Check sheet for the modelled part. Datum: model origin and axes. Units: mm. A direction names the side the tool comes from. Round coordinates to 2 decimals unless told otherwise and drop trailing zeros. Loops run counter-clockwise (first coordinate to the right, second up) from the corner with the lowest first, then second, coordinate; pieces in that order, holes last. Notation, with made-up numbers: (-8, -11) - (45, -11) arc R20 ccw to (45, -5) - close; hole circle Ø3 at (10.5, 30). An arc over 180 degrees is marked (long way). Put each result on its own line as item: value.
```python
from build123d import *

# Parameters (mm, degrees)
F0_R      = 17.4625
F0_R_2    = 4.7625
F1_DEPTH  = 4.7752
F2_R      = 7.9375
F2_R_2    = 4.7625
F3_DEPTH  = 6.35
F5_R      = 1.5875
F6_DEPTH  = 4.7762
F8_R      = 1.4224
F9_DEPTH  = 5.08
F11_R     = 1.4224
F12_DEPTH = 5.08


with BuildPart() as f1:
    # F0 (on Front) → F1 (new body)
    with BuildSketch(Plane.XZ):
        Circle(F0_R)
        Circle(F0_R_2, mode=Mode.SUBTRACT)
    extrude(amount=F1_DEPTH)

    # F2 (on face) → F3 (join)
    with BuildSketch(Plane.XZ.offset(4.7752)):
        Circle(F2_R)
        Circle(F2_R_2, mode=Mode.SUBTRACT)
    extrude(amount=F3_DEPTH)

    # F5 (on face) → F6 (cut, through all)
    with BuildSketch(Plane.XZ.offset(4.7752)):
        with Locations((0, 13.97)):
            Circle(F5_R)
    extrude(amount=-F6_DEPTH, mode=Mode.SUBTRACT)

    # F8 (on offset) → F9 (cut)
    with BuildSketch(Plane.XY.offset(7.9375)):
        with Locations((0, -7.9502)):
            Circle(F8_R)
    extrude(amount=-F9_DEPTH, mode=Mode.SUBTRACT)

    # F11 (on offset) → F12 (cut)
    with BuildSketch(Plane.YZ.offset(7.9375)):
        with Locations((-7.9502, 0)):
            Circle(F11_R)
    extrude(amount=-F12_DEPTH, mode=Mode.SUBTRACT)


solid = f1.part
```
Item 1: Section check A-A on z = 0. Enter the section's corners in (x, y).
Filled sheet:
outline: (-17.46, -4.78) - (-7.94, -4.78) - (-7.94, -11.13) - (-4.76, -11.13) - (-4.76, 0) - (-17.46, 0) - close; (4.76, -11.13) - (7.94, -11.13) - (7.94, -9.37) - (4.76, -9.37) - close; (4.76, -6.53) - (7.94, -6.53) - (7.94, -4.78) - (17.46, -4.78) - (17.46, 0) - (4.76, 0) - close
Item 2: Section check D-D on z = 13.97. Enter the section's corners in (x, y).
Filled sheet:
outline: (-10.48, -4.78) - (-1.59, -4.78) - (-1.59, 0) - (-10.48, 0) - close; (1.59, -4.78) - (10.48, -4.78) - (10.48, 0) - (1.59, 0) - close
Item 3: Release check for a two-part mould opening along X. For faces 4 (the cylindrical face through (-1.03, -5.48, -4.65)), 5 (the flat face through (0, -11.125, -5)), 6 (the cylindrical face through (-1.72, -7.91, -7.75)) record: +X half, -X half, draft (parallel to the pull), parting line (faces both ways), or undercut.
Filled sheet:
face 4: undercut
face 5: draft
face 6: parting line
Item 4: Tool access check on faces 1 (the flat face through (4, -4.775, -8)), 2 (the cylindrical face through (1.314, -8.495, 6.262)), 3 (the cylindrical face through (6.265, -6.593, 0.427)). Record the directions out of +Z, -Z, +X, -X, +Y, -Y that give a thin tool (end or side, any length) a straight path to the whole face; none if there is none.
Filled sheet:
face 1: -Y
face 2: +Z
face 3: +X
Item 5: Thickness scan on line 1 (Z direction, x = 0, y = -2.55); line 2 (Z direction, x = 0, y = -5); line 3 (Y direction, x = 0, z = 5.4). Record the ranges inside material, lowest first. Write a range as from..to.
Filled sheet:
line 1: -17.46..-4.76, 4.76..12.38, 15.56..17.46
line 2: -7.94..-4.76, 4.76..7.94
line 3: -11.13..-9.37, -6.53..0
Item 6: Go/stop test with flat-tipped pins: pin 1 (3 mm diameter, centred on x = 10.5, z = 6, fed in from -Y); pin 2 (3 mm diameter, centred on y = -4.5, z = 8, fed in from -X); pin 3 (6 mm diameter, centred on x = 13, y = -6.5, fed in from +Z); pin 4 (10.5 mm diameter, centred on x = -0.5, z = 1.5, fed in from -Y). Record where each tip stops, or that it passes through.
Filled sheet:
pin 1: y = -4.78
pin 2: x = -16.21
pin 3: z = 13.92
pin 4: y = -11.13
Item 7: Section check B-B on x = 2. Enter the section's corners in (y, z), then the cut area to 3 significant figures.
Filled sheet:
outline: (-11.13, -7.68) - (-4.78, -7.68) - (-4.78, -17.35) - (0, -17.35) - (0, -4.32) - (-11.13, -4.32) - close; (-11.13, 4.32) - (0, 4.32) - (0, 17.35) - (-4.78, 17.35) - (-4.78, 7.68) - (-11.13, 7.68) - close
area: 167 mm²
Item 8: Section check C-C on y = -8.5. Enter the section's corners in (x, z) (1 decimal).
Filled sheet:
outline: (-1.3, 4.6) - (-1.3, 7.8) arc R7.9 ccw (long way) to (7.8, -1.3) - (4.6, -1.3) arc R4.8 cw (long way) to start; (1.3, 4.6) arc R4.8 cw to (4.6, 1.3) - (7.8, 1.3) arc R7.9 ccw to (1.3, 7.8) - close
